Autodesk Fusion 360 part; units mm, degrees
sketch "Sketch1" plane through (0, 0, 0) normal (0, 1, 0) x (1, 0, 0)
  line L0 (0, 0) -> (90, 0)
  line L1 (90, 0) -> (90, -5)
  line L2 (90, -5) -> (0, -5)
  line L3 (0, -5) -> (0, 0)
  dimension "d1" = 90
  dimension "d2" = 5
extrude "Extrude1" add sketch "Sketch1" along normal blind 10
extrude "Extrude2" add 1 faces at (30, 10, 1.6667) along direction (0, 1, 0) blind 5
extrude "Extrude3" add 1 faces at (30, 15, 1.6667) along direction (0, 1, 0) blind 5
sketch "Sketch2" plane through (0, 0, 5) normal (0, 0, 1) x (1, 0, 0)
  line L0 (0, 0) -> (90, 0)
  line L1 (90, 0) -> (90, 20)
  line L2 (90, 20) -> (0, 20)
  line L3 (0, 20) -> (0, 0)
  line L4 (0, 0) -> (15.42, 0)
  line L5 (15.42, 20) -> (0, 20)
  line L6 (15.42, 20) -> (15.42, 0)
  line L7 (0, 0) -> (0, 20)
  line L8 (90, 0) -> (74.58, 0)
  line L9 (74.58, 0) -> (74.58, 20)
  line L10 (74.58, 20) -> (90, 20)
  line L11 (90, 0) -> (90, 20)
  dimension "d9" = 15.42
  dimension "d10" = 15.42
extrude "Extrude4" add sketch "Sketch2" along normal blind 10 contours L0 L2 L3 L4 L5 L6 L7 | L0 L1 L2 L8 L9 L10 L11
sketch "Sketch3" plane through (0, 0, 15) normal (0, 0, 1) x (1, 0, 0)
  line L0 (15.42, 20) -> (0, 20)
  line L1 (0, 20) -> (0, 0)
  line L2 (0, 0) -> (15.42, 0)
  line L3 (15.42, 0) -> (15.42, 20)
  circle A0 centre (7.2922, 9.4249) radius 5
  dimension "d13" = 10
sketch "Sketch4" plane through (0, 0, 15) normal (0, 0, 1) x (1, 0, 0)
  line L0 (74.58, 0) -> (90, 0)
  line L1 (90, 0) -> (90, 20)
  line L2 (90, 20) -> (74.58, 20)
  line L3 (74.58, 20) -> (74.58, 0)
  circle A0 centre (82.29, 10.052) radius 5
  dimension "d14" = 10
extrude "Extrude5" add sketch "Sketch3" sketch "Sketch4" along normal blind 40 contours A0 of sketch 2 contours A0
thread "Thread1"
thread "Thread2"
hole "Hole1" at (46.3648, 9.7949, 5) direction (0, 0, -1) diameter 10 depth 20 tip angle 118
Part model, mm, in its own coordinate system. A direction names the side the tool comes from. Round coordinates to 2 decimals unless told otherwise and drop trailing zeros. Loops run counter-clockwise (first coordinate to the right, second up) from the corner with the lowest first, then second, coordinate; pieces in that order, holes last. Notation, with made-up numbers: (42.5, 44.5) -> (46.5, 44.5) arc R33 cw to (46.5, 83.5) -> close; hole circle Ø8 at (63, 54). An arc over 180 degrees is marked (long way). Use CSV: the item, a comma, the result in double quotes. Start each with the question number.
1) Cut at C-C, the plane x = 82.29. Write the cut outline in (y, z).
2) Drop flat-ended pins along their axis: P1, Ø2, axis at y = 15.5, z = 36, coming from the +X side; P2, Ø12, axis at y = 7, z = 47, coming from the +X side; P3, Ø2, axis at x = 67.5, y = 5.5, coming from the +Z side. Give the stop position or say it passes through.
3) Cut at B-B, the plane y = 8.5. Write the cut outline in (x, z), plus the area to 3 significant figures.
4) Which spindle directions (+Z, -Z, +X, -X, +Y, -Y) get a long thin tool onto all of the face, cutting with end or side? Do faces 1 (the cylindrical face through (12.06, 7.92, 34.72)), 2 (the cylindrical face through (42.149, 7.107, 2.465)), 3 (the flat face through (52, 10, 5)). Say none if no direction does.
5) Wall check: L1, parallel to X at y = 16.5, z = 14.5; L2, parallel to Z at x = 41, y = 18; L3, parallel to Z at x = 11, y = 14.5. Give the ranges that are in metal, low to high. Write a range as [from, to].
6) Cut at A-A, the plane z = 10. Write the cut outline in (x, y), plus the area to 3 significant figures.
7) Pull direction X, two halves, no side cores. Call faces 4 (the flat face through (90, 10, 7)), 5 (the cylindrical face through (86.909, 11.967, 34.72)), 6 (the flat face through (0, 10, 8)): +X half, -X half, draft (parallel to the pull), parting line (faces both ways), or undercut.
8) Cut at D-D, the plane y = 3. Write the cut outline in (x, z).
Determined:
1,outline,"(0, 0) -> (20, 0) -> (20, 15) -> (15.05, 15) -> (15.05, 55) -> (5.05, 55) -> (5.05, 15) -> (0, 15) -> close"
2,P1,"stops at x = 84.57"
2,P2,"stops at x = 87.29"
2,P3,"stops at z = 5"
3,outline,"(0, 0) -> (41.54, 0) -> (41.54, 5) -> (15.42, 5) -> (15.42, 15) -> (12.21, 15) -> (12.21, 55) -> (2.38, 55) -> (2.38, 15) -> (0, 15) -> close; (51.19, 0) -> (90, 0) -> (90, 15) -> (87.04, 15) -> (87.04, 55) -> (77.54, 55) -> (77.54, 15) -> (74.58, 15) -> (74.58, 5) -> (51.19, 5) -> close"
3,area,"1,480 mm2"
4,face 1,"+Z"
4,face 2,"+Z, -Z"
4,face 3,"+Z, +Y, -Y"
5,L1,"x = [0, 15.42], [74.58, 90]"
5,L2,"z = [0, 5]"
5,L3,"z = [0, 15]"
6,outline,"(0, 0) -> (15.42, 0) -> (15.42, 20) -> (0, 20) -> close; (74.58, 0) -> (90, 0) -> (90, 20) -> (74.58, 20) -> close"
6,area,"617 mm2"
7,face 4,"+X half"
7,face 5,"undercut"
7,face 6,"-X half"
8,outline,"(0, 0) -> (90, 0) -> (90, 15) -> (74.58, 15) -> (74.58, 5) -> (15.42, 5) -> (15.42, 15) -> (0, 15) -> close"
